Check sheet for the drawn part. Datum: minimum x, y, z corner. Units: mm. Round coordinates to 2 decimals unless told otherwise and drop trailing zeros. Loops run counter-clockwise (first coordinate to the right, second up) from the corner with the lowest first, then second, coordinate; pieces in that order, holes last.
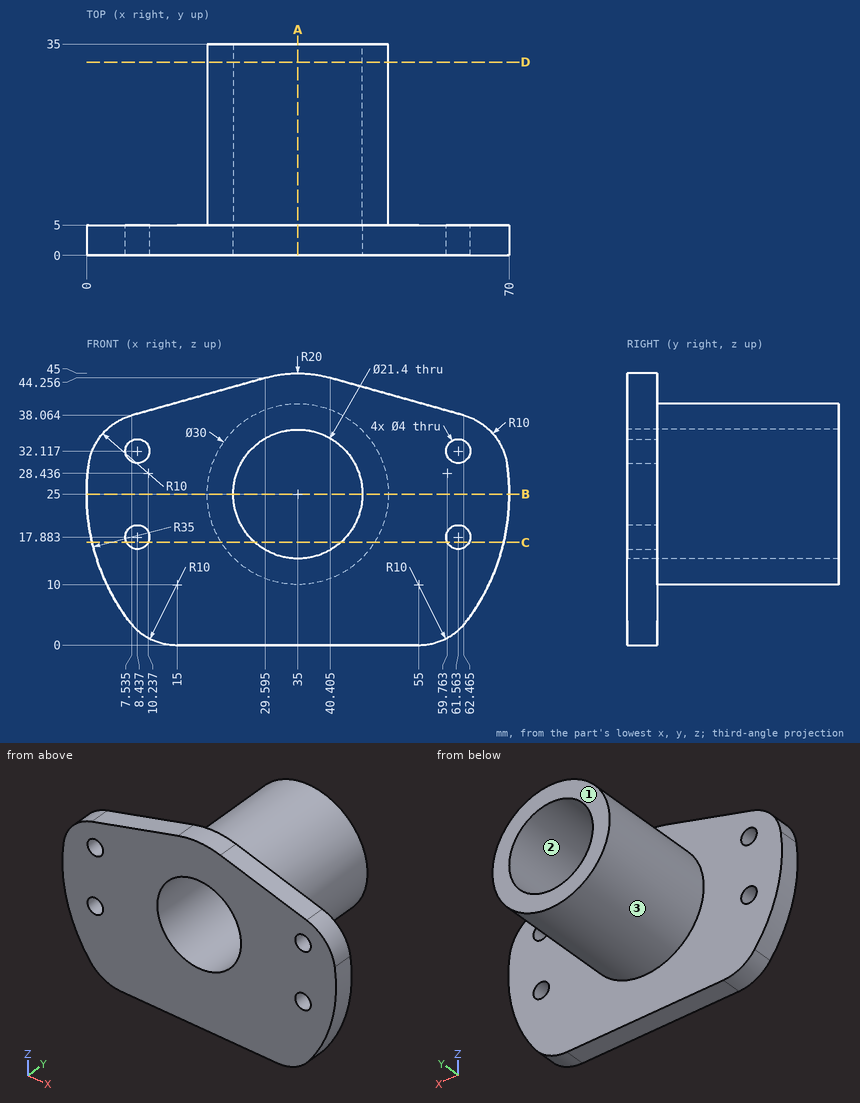
1) Sectioned sample at C-C, the plane z = 17. Record the cut outline in (x, y) (1 decimal).
Report:
outline: (0.9, 0) - (6.6, 0) - (6.6, 5) - (0.9, 5) - close; (10.2, 0) - (27.9, 0) - (27.9, 35) - (22.3, 35) - (22.3, 5) - (10.2, 5) - close; (42.1, 0) - (59.8, 0) - (59.8, 5) - (47.7, 5) - (47.7, 35) - (42.1, 35) - close; (63.4, 0) - (69.1, 0) - (69.1, 5) - (63.4, 5) - close
2) Sectioned sample at A-A, the plane x = 35. Record the cut outline in (y, z).
Report:
outline: (0, 0) - (5, 0) - (5, 10) - (35, 10) - (35, 14.3) - (0, 14.3) - close; (0, 35.7) - (35, 35.7) - (35, 40) - (5, 40) - (5, 45) - (0, 45) - close
3) Sectioned sample at D-D, the plane y = 32. Record the cut outline in (x, z).
Report:
outline: circle Ø30 at (35, 25); hole circle Ø21.4 at (35, 25)
4) Scan lines: line 1 along Z through (x, y) = (35, 26.5); line 2 along Y through (x, z) = (18.5, 23); line 3 along X through (y, z) = (21, 24.5). Record each from-to range of solid material in increasing order.
Report:
line 1: z = 10 to 14.3, 35.7 to 40
line 2: y = 0 to 5
line 3: x = 20.01 to 24.31, 45.69 to 49.99
5) Sectioned sample at B-B, the plane z = 25. Record the cut outline in (x, y), then the cut area to 3 significant figures.
Report:
outline: (0, 0) - (24.3, 0) - (24.3, 35) - (20, 35) - (20, 5) - (0, 5) - close; (45.7, 0) - (70, 0) - (70, 5) - (50, 5) - (50, 35) - (45.7, 35) - close
area: 501 mm2
6) Mould release check, pull along Z, two halves, no side actions. Record for the marked faces 1, 2 and 3: +Z half, -Z half, draft (parallel to the pull), parting line (faces both ways), or undercut.
Report:
face 1: draft
face 2: undercut
face 3: parting line
7) Gauge pin test, flat ends, axial feed: pin 1 (5 mm diameter, centred on y = 26, z = 12.5, fed in from +X); pin 2 (4 mm diameter, centred on x = 29, y = 20, fed in from -Z); pin 3 (3.5 mm diameter, centred on x = 8.44, z = 17.88, fed in from +Y); pin 4 (10 mm diameter, centred on x = 9, z = 40, fed in from +Y). Record the tip position at first contact, or that the pin passes through.
Report:
pin 1: stops at x = 46.18
pin 2: stops at z = 10.54
pin 3: passes through
pin 4: stops at y = 5
